Geometry check sheet. Reference: the model listing, model coordinates, mm. Face numbers are marked on the shaded views. A direction names the side the tool comes from. Give positions to 0.01 mm unless a question says otherwise; leave off trailing zeros. Loops run counter-clockwise (first coordinate to the right, second up) from the corner with the lowest first, then second, coordinate; pieces in that order, holes last. Notation, with made-up numbers: (14.5, 25) - (23.5, 25) arc R11 ccw to (23.5, 29) - close; hole circle Ø7 at (-7.75, -38.75). An arc over 180 degrees is marked (long way). Use a Markdown table: item, result. Add a question column.
1. Cross-section at A-A on y = 7.75. Enter the section's corners in (x, z), and give its area (3 significant figures).
2. Draft check along X on the marked faces 1, 2 and 3. Enter one of: pulls with the +X half, pulls with the -X half, needs draft (parallel to the pull), parting line crosses it, or undercut.
3. Cross-section at D-D on z = 7.5. Enter the section's corners in (x, y).
4. Set-up check for the marked faces 4, 5, 6 and 7: record each of +Z, -Z, +X, -X, +Y, -Y from which the full face is reachable in a straight line by a thin tool's end or side.
5. Cross-section at C-C on y = 18.75. Enter the section's corners in (x, z).
6. Material ranges on L1, parallel to X at y = 15.5, z = 9; L2, parallel to Y at x = -8, z = 18; L3, parallel to Z at x = -31, y = 12, recorded low to high.
7. Cross-section at B-B on x = -33.5. Enter the section's corners in (y, z), and give its area (3 significant figures).
8. Depth check by flat-ended pin: P1, Ø1.9, axis at y = 17, z = 19, coming from the +X side; P2, Ø3.5, axis at x = -19.5, z = 1.5, coming from the -Y side; P3, Ø9, axis at y = 13, z = 11, coming from the -X side. Enter the tip coordinate at first touch or a pass-through.
from build123d import *

# Parameters (mm, degrees)
F2_DEPTH     = 35
F3_DEPTH     = 3
F4_DEPTH     = 25
F5_R         = 4.99999
F6_T1_DEPTH  = 35
F6_T3_DEPTH  = 35
F6_T8_DEPTH  = 60
F6_T13_DEPTH = 60
F6_T15_DEPTH = 43.4564392374
F6_T20_DEPTH = 60
F6_T25_DEPTH = 60
F6_T27_DEPTH = 43.4564392374
F7_T1_DEPTH  = 6.417424305
F7_T3_DEPTH  = 30
F7_T6_ANGLE  = 89.9999999974
F7_T8_ANGLE  = 89.9999999974
F7_T10_ANGLE = 209.6926070845
F7_T12_ANGLE = 209.6926070845


# Not quite as in the source:
# - a fillet or chamfer that OpenCascade refuses, or shapes differently, is made with other operations: its cross-section is extruded or revolved along the edge and cut away or added
# - a fillet or chamfer is up to 0.001 mm smaller than in the source, because OpenCascade refuses the exact size


with BuildPart() as f2:
    # F0 (on Top) → F2 (new body)
    with BuildSketch(Plane.XY):
        Polygon((20, 26), (0, 26), (-20, 26), (-20, 22), (-20, 10), (-17, 10), (-17, 23), (0, 23), (17, 23), (17, 10), (20, 10), (20, 22), align=None)
    extrude(amount=F2_DEPTH)

    # F0 (on Top) → F3 (join)
    with BuildSketch(Plane.XY):
        Polygon((-20, 10), (-20, 22), (-37.5, 22), (-37.5, 0), (-27.5, 0), (-27.5, 10), align=None)
        Polygon((37.5, 22), (20, 22), (20, 10), (27.5, 10), (27.5, 0), (37.5, 0), align=None)
    extrude(amount=F3_DEPTH)

    # F1 (on Top) → F4 (cut)
    with BuildSketch(Plane.XY):
        with BuildLine():
            Line((35, 3.8767794613), (35, 15.8767794613))
            ThreePointArc((35, 15.8767794613), (33.5, 17.3767794613), (32, 15.8767794613))
            Line((32, 15.8767794613), (32, 3.8767794613))
            ThreePointArc((32, 3.8767794613), (33.5, 2.3767794613), (35, 3.8767794613))
        make_face()
        with BuildLine():
            ThreePointArc((-32, 15.8767794613), (-33.5, 17.3767794613), (-35, 15.8767794613))
            Line((-35, 15.8767794613), (-35, 3.8767794613))
            ThreePointArc((-35, 3.8767794613), (-33.5, 2.3767794613), (-32, 3.8767794613))
            Line((-32, 3.8767794613), (-32, 15.8767794613))
        make_face()
    extrude(amount=F4_DEPTH, mode=Mode.SUBTRACT)

    # F5 (radius 5 in the source; OpenCascade refuses exactly that, so slightly less here)
    f5_edges = [f2.edges().sort_by_distance(p)[0] for p in [
        (-37.5, 0, 1.5),
        (-27.5, 0, 1.5),
        (-37.5, 22, 1.5),
        (37.5, 22, 1.5),
        (37.5, 0, 1.5),
        (27.5, 0, 1.5),
        (27.5, 10, 1.5),
        (-27.5, 10, 1.5),
    ]]
    fillet(f5_edges, radius=F5_R)

    # F6: fillet of radius 5 on 6 edges, made by hand

    # F6_s2 → F6_t1 (join)
    with BuildSketch(Plane.XY):
        with BuildLine():
            ThreePointArc((17, 18), (15.5355339059, 21.5355339059), (12, 23))
            Line((12, 23), (17, 23))
            Line((17, 23), (17, 18))
        make_face()
    extrude(amount=F6_T1_DEPTH)

    # F6_s4 → F6_t3 (join)
    with BuildSketch(Plane.XY):
        with BuildLine():
            ThreePointArc((-12, 23), (-15.5355339059, 21.5355339059), (-17, 18))
            Line((-17, 18), (-17, 23))
            Line((-17, 23), (-12, 23))
        make_face()
    extrude(amount=F6_T3_DEPTH)


with BuildPart() as f6_tool6:
    # F6_s7 → F6_t8 (new body)
    with BuildSketch(Plane.XY.offset(-12.5)):
        with BuildLine():
            ThreePointArc((20, 21), (18.5355339059, 24.5355339059), (15, 26))
            Line((15, 26), (20, 26))
            Line((20, 26), (20, 21))
        make_face()
    extrude(amount=F6_T8_DEPTH)

    split(bisect_by=Plane.XZ.offset(-22), keep=Keep.BOTTOM)


with BuildPart() as f2_1:
    add(f2.part)

    # F6_t5: cut F6_tool6
    add(f6_tool6.part, mode=Mode.SUBTRACT)


with BuildPart() as f6_tool11:
    # F6_s12 → F6_t13 (new body)
    with BuildSketch(Plane.XY.offset(-12.5)):
        with BuildLine():
            ThreePointArc((20, 21), (18.5355339059, 24.5355339059), (15, 26))
            Line((15, 26), (20, 26))
            Line((20, 26), (20, 21))
        make_face()
    extrude(amount=F6_T13_DEPTH)

    split(bisect_by=Plane.XY.offset(3), keep=Keep.TOP)


with BuildPart() as f2_2:
    add(f2_1.part)

    # F6_t10: cut F6_tool11
    add(f6_tool11.part, mode=Mode.SUBTRACT)

    # F6_s16 → F6_t15 (cut)
    with BuildSketch(Plane.XY.offset(3)):
        with BuildLine():
            ThreePointArc((20, 14.582575695), (19.1833001327, 11.8439629074), (17, 10))
            Line((17, 10), (20, 10))
            Line((20, 10), (20, 14.582575695))
        make_face()
    extrude(amount=F6_T15_DEPTH, mode=Mode.SUBTRACT)


with BuildPart() as f6_tool18:
    # F6_s19 → F6_t20 (new body)
    with BuildSketch(Plane.XY.offset(-12.5)):
        with BuildLine():
            ThreePointArc((-20, 21), (-18.5355339059, 24.5355339059), (-15, 26))
            Line((-15, 26), (-20, 26))
            Line((-20, 26), (-20, 21))
        make_face()
    extrude(amount=F6_T20_DEPTH)

    split(bisect_by=Plane.XZ.offset(-22), keep=Keep.BOTTOM)


with BuildPart() as f2_3:
    add(f2_2.part)

    # F6_t17: cut F6_tool18
    add(f6_tool18.part, mode=Mode.SUBTRACT)


with BuildPart() as f6_tool23:
    # F6_s24 → F6_t25 (new body)
    with BuildSketch(Plane.XY.offset(-12.5)):
        with BuildLine():
            ThreePointArc((-20, 21), (-18.5355339059, 24.5355339059), (-15, 26))
            Line((-15, 26), (-20, 26))
            Line((-20, 26), (-20, 21))
        make_face()
    extrude(amount=F6_T25_DEPTH)

    split(bisect_by=Plane.XY.offset(3), keep=Keep.TOP)


with BuildPart() as f2_4:
    add(f2_3.part)

    # F6_t22: cut F6_tool23
    add(f6_tool23.part, mode=Mode.SUBTRACT)

    # F6_s28 → F6_t27 (cut)
    with BuildSketch(Plane.XY.offset(3)):
        with BuildLine():
            ThreePointArc((-20, 14.582575695), (-19.1833001327, 11.8439629074), (-17, 10))
            Line((-17, 10), (-20, 10))
            Line((-20, 10), (-20, 14.582575695))
        make_face()
    extrude(amount=F6_T27_DEPTH, mode=Mode.SUBTRACT)

    # F7: fillet of radius 5 on 3 edges, made by hand

    # F7_s2 → F7_t1 (cut)
    with BuildSketch(Plane.XZ.offset(-21)):
        with BuildLine():
            ThreePointArc((-15, 35), (-18.5355339059, 33.5355339059), (-20, 30))
            Line((-20, 30), (-20, 35))
            Line((-20, 35), (-15, 35))
        make_face()
        with BuildLine():
            ThreePointArc((15, 35), (18.5355339059, 33.5355339059), (20, 30))
            Line((20, 30), (20, 35))
            Line((20, 35), (15, 35))
        make_face()
    extrude(amount=F7_T1_DEPTH, mode=Mode.SUBTRACT)

    # F7_s4 → F7_t3 (cut)
    with BuildSketch(Plane.YZ.offset(-15)):
        with BuildLine():
            ThreePointArc((21, 35), (24.5355339059, 33.5355339059), (26, 30))
            Line((26, 30), (26, 35))
            Line((26, 35), (21, 35))
        make_face()
    extrude(amount=F7_T3_DEPTH, mode=Mode.SUBTRACT)

    # F7_s5 → F7_t6 (revolve, cut)
    with BuildSketch(Plane.YZ.offset(14.9999999999)):
        with BuildLine():
            ThreePointArc((21, 35), (24.5355339059, 33.5355339059), (26, 30))
            Line((26, 30), (26, 35))
            Line((26, 35), (21, 35))
        make_face()
    revolve(axis=Axis((14.9999999999, 20.9999999999, 35), (0, 0, -1)), revolution_arc=F7_T6_ANGLE, mode=Mode.SUBTRACT)

    # F7_s7 → F7_t8 (revolve, cut)
    with BuildSketch(Plane.XZ.offset(-20.9999999999)):
        with BuildLine():
            ThreePointArc((-15, 35), (-18.5355339059, 33.5355339059), (-20, 30))
            Line((-20, 30), (-20, 35))
            Line((-20, 35), (-15, 35))
        make_face()
    revolve(axis=Axis((-14.9999999999, 20.9999999999, 35), (0, 0, -1)), revolution_arc=F7_T8_ANGLE, mode=Mode.SUBTRACT)

    # F7_s9 → F7_t10 (revolve, cut)
    with BuildSketch(Plane.XZ.offset(-14.5825756948)):
        with BuildLine():
            ThreePointArc((20, 30), (18.5355339059, 33.5355339059), (15, 35))
            Line((15, 35), (20, 35))
            Line((20, 35), (20, 30))
        make_face()
    revolve(axis=Axis((15.0000000002, 14.5825756948, 35), (0, 0, -1)), revolution_arc=F7_T10_ANGLE, mode=Mode.SUBTRACT)

    # F7_s11 → F7_t12 (revolve, cut)
    with BuildSketch(Plane(origin=(-9.9554834358, 17.4590545428, 0), x_dir=(0, 0, 1), z_dir=(-0.4953465841, 0.8686954366, 0))):
        with BuildLine():
            ThreePointArc((35, -5.8070024913), (33.5355339059, -2.2714685854), (30, -0.8070024913))
            Line((30, -0.8070024913), (35, -0.8070024913))
            Line((35, -0.8070024913), (35, -5.8070024913))
        make_face()
    revolve(axis=Axis((-15.0000000002, 14.5825756948, 35), (0, 0, -1)), revolution_arc=F7_T12_ANGLE, mode=Mode.SUBTRACT)


solid = f2_4.part
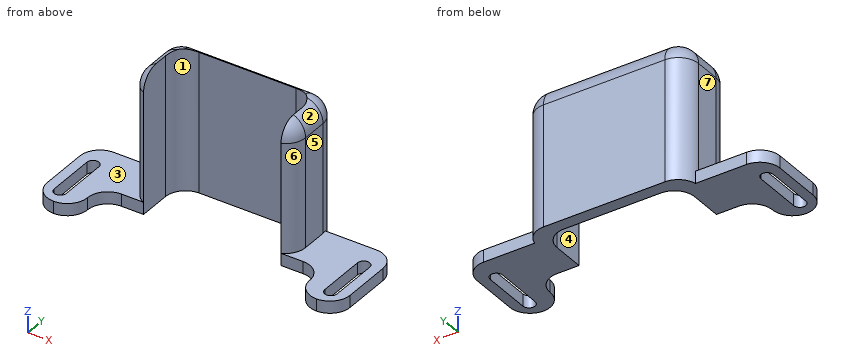
Values found:
| question | item | result |
|---|---|---|
| 1 | outline | (-37.5, 0) - (-35, 0) - (-35, 3) - (-37.5, 3) - close; (-32, 0) - (-26.68, 0) - (-26.68, 3) - (-32, 3) - close; (26.68, 0) - (32, 0) - (32, 3) - (26.68, 3) - close; (35, 0) - (37.5, 0) - (37.5, 3) - (35, 3) - close |
| 1 | area | 46.9 mm2 |
| 2 | face 1 | undercut |
| 2 | face 2 | pulls with the +X half |
| 2 | face 3 | needs draft |
| 3 | outline | (-20, 14.58) arc R5 ccw to (-17, 10) - (-17, 18) arc R5 cw to (-12, 23) - (12, 23) arc R5 cw to (17, 18) - (17, 10) arc R5 ccw to (20, 14.58) - (20, 21) arc R5 ccw to (15, 26) - (-15, 26) arc R5 ccw to (-20, 21) - close |
| 4 | face 4 | +Z, -Z, -Y |
| 4 | face 5 | +Z, +X, +Y, -Y |
| 4 | face 6 | +Z, +X, -Y |
| 4 | face 7 | +Z, -X, +Y, -Y |
| 5 | outline | (-37.18, 0) - (-16.94, 0) - (-16.94, 34.61) arc R5 ccw to (-20, 30) - (-20, 3) - (-37.18, 3) - close; (16.94, 0) - (37.18, 0) - (37.18, 3) - (20, 3) - (20, 30) arc R5 ccw to (16.94, 34.61) - close |
| 6 | L1 | x = -20 to -17, 17 to 20 |
| 6 | L2 | y = 23 to 26 |
| 6 | L3 | z = 0 to 3 |
| 7 | outline | (0.1, 0) - (2.38, 0) - (2.38, 3) - (0.1, 3) - close; (17.38, 0) - (21.9, 0) - (21.9, 3) - (17.38, 3) - close |
| 7 | area | 20.4 mm2 |
| 8 | P1 | stops at x = 20 |
| 8 | P2 | stops at y = 10 |
| 8 | P3 | stops at x = -20 |
